from build123d import *

# Parameters (mm, degrees)
SKETCH_1_R          = 1.3
SKETCH_1_R_2        = 3
SKETCH_1_R_3        = 3.1
EXTRUDE_1_DEPTH     = 18
CUT_EXTRUDE_1_DEPTH = 39.778149269


with BuildPart() as part:
    # ｽｹｯﾁ1 → ﾎﾞｽ - 押し出し1 (new body)
    with BuildSketch(Plane.XY):
        with BuildLine():
            ThreePointArc((11.520520871, 18.842793666), (9.949769241, 24.020867845), (5.177628747, 21.470105609))
            ThreePointArc((5.177628747, 21.470105609), (0, 17.220935509), (-5.177628747, 21.470105609))
            ThreePointArc((-5.177628747, 21.470105609), (-9.949769241, 24.020867845), (-11.520520871, 18.842793666))
            ThreePointArc((-11.520520871, 18.842793666), (-12.177040277, 12.177040277), (-18.842793666, 11.520520871))
            ThreePointArc((-18.842793666, 11.520520871), (-24.020867845, 9.949769241), (-21.470105609, 5.177628747))
            ThreePointArc((-21.470105609, 5.177628747), (-17.220935509, 0), (-21.470105609, -5.177628747))
            ThreePointArc((-21.470105609, -5.177628747), (-24.020867845, -9.949769241), (-18.842793666, -11.520520871))
            ThreePointArc((-18.842793666, -11.520520871), (-12.177040277, -12.177040277), (-11.520520871, -18.842793666))
            ThreePointArc((-11.520520871, -18.842793666), (-9.949769241, -24.020867845), (-5.177628747, -21.470105609))
            ThreePointArc((-5.177628747, -21.470105609), (0, -17.220935509), (5.177628747, -21.470105609))
            ThreePointArc((5.177628747, -21.470105609), (9.949769241, -24.020867845), (11.520520871, -18.842793666))
            ThreePointArc((11.520520871, -18.842793666), (12.177040277, -12.177040277), (18.842793666, -11.520520871))
            ThreePointArc((18.842793666, -11.520520871), (24.020867845, -9.949769241), (21.470105609, -5.177628747))
            ThreePointArc((21.470105609, -5.177628747), (17.220935509, 0), (21.470105609, 5.177628747))
            ThreePointArc((21.470105609, 5.177628747), (24.020867845, 9.949769241), (18.842793666, 11.520520871))
            ThreePointArc((18.842793666, 11.520520871), (12.177040277, 12.177040277), (11.520520871, 18.842793666))
        make_face()
        with Locations((8.610377228, 20.787289482)):
            Circle(SKETCH_1_R, mode=Mode.SUBTRACT)
        with Locations((20.787289482, 8.610377228)):
            Circle(SKETCH_1_R, mode=Mode.SUBTRACT)
        with Locations((20.787289482, -8.610377228)):
            Circle(SKETCH_1_R, mode=Mode.SUBTRACT)
        with Locations((8.610377228, -20.787289482)):
            Circle(SKETCH_1_R, mode=Mode.SUBTRACT)
        with Locations((-8.610377228, -20.787289482)):
            Circle(SKETCH_1_R, mode=Mode.SUBTRACT)
        with Locations((-20.787289482, -8.610377228)):
            Circle(SKETCH_1_R, mode=Mode.SUBTRACT)
        with Locations((-20.787289482, 8.610377228)):
            Circle(SKETCH_1_R, mode=Mode.SUBTRACT)
        with Locations((-8.610377228, 20.787289482)):
            Circle(SKETCH_1_R, mode=Mode.SUBTRACT)
        with Locations((8.838834765, 8.838834765)):
            Circle(SKETCH_1_R, mode=Mode.SUBTRACT)
        with Locations((8.838834765, -8.838834765)):
            Circle(SKETCH_1_R, mode=Mode.SUBTRACT)
        with Locations((-8.838834765, -8.838834765)):
            Circle(SKETCH_1_R, mode=Mode.SUBTRACT)
        with Locations((-8.838834765, 8.838834765)):
            Circle(SKETCH_1_R, mode=Mode.SUBTRACT)
        with Locations((0, 6.5)):
            Circle(SKETCH_1_R, mode=Mode.SUBTRACT)
        with Locations((6.5, 0)):
            Circle(SKETCH_1_R, mode=Mode.SUBTRACT)
        with Locations((0, -6.5)):
            Circle(SKETCH_1_R, mode=Mode.SUBTRACT)
        with Locations((-6.5, 0)):
            Circle(SKETCH_1_R, mode=Mode.SUBTRACT)
        with Locations((0, 12.5)):
            Circle(SKETCH_1_R_2, mode=Mode.SUBTRACT)
        with Locations((12.5, 0)):
            Circle(SKETCH_1_R_2, mode=Mode.SUBTRACT)
        with Locations((0, -12.5)):
            Circle(SKETCH_1_R_2, mode=Mode.SUBTRACT)
        with Locations((-12.5, 0)):
            Circle(SKETCH_1_R_2, mode=Mode.SUBTRACT)
        Circle(SKETCH_1_R_3, mode=Mode.SUBTRACT)
    extrude(amount=EXTRUDE_1_DEPTH)

    # ｽｹｯﾁ2 → ｶｯﾄ - 押し出し1 (cut, through all)
    with BuildSketch(Plane.XY.offset(18)):
        with BuildLine():
            ThreePointArc((-15.5, 6e-09), (-12.499999997, 3), (-9.5, 0))
            ThreePointArc((-9.5, 0), (-9.355673654, 1.649657688), (-8.927079897, 3.249191362))
            ThreePointArc((-8.927079897, 3.249191362), (-10.72009733, 7.094329654), (-14.565235622, 5.301312222))
            ThreePointArc((-14.565235622, 5.301312222), (-15.264520171, 2.691546757), (-15.5, 6e-09))
        make_face()
        with BuildLine():
            ThreePointArc((-14.565235622, -5.301312222), (-10.72009733, -7.094329654), (-8.927079897, -3.249191362))
            ThreePointArc((-8.927079897, -3.249191362), (-9.355673654, -1.649657688), (-9.5, 0))
            ThreePointArc((-9.5, 0), (-12.500000003, -3), (-15.5, 6e-09))
            ThreePointArc((-15.5, 6e-09), (-15.264520172, -2.691546751), (-14.565235622, -5.301312222))
        make_face()
        with BuildLine():
            ThreePointArc((5.301312222, -14.565235622), (7.094329654, -10.72009733), (3.249191362, -8.927079897))
            ThreePointArc((3.249191362, -8.927079897), (1.649657689, -9.355673653), (3e-09, -9.5))
            ThreePointArc((3e-09, -9.5), (2.121320344, -10.378679657), (3, -12.5))
            ThreePointArc((3, -12.5), (2.121320344, -14.621320343), (1e-09, -15.5))
            ThreePointArc((1e-09, -15.5), (2.691546754, -15.264520172), (5.301312222, -14.565235622))
        make_face()
        with BuildLine():
            ThreePointArc((1e-09, -15.5), (-3, -12.499999999), (3e-09, -9.5))
            ThreePointArc((3e-09, -9.5), (-1.649657687, -9.355673654), (-3.249191362, -8.927079897))
            ThreePointArc((-3.249191362, -8.927079897), (-7.094329654, -10.72009733), (-5.301312222, -14.565235622))
            ThreePointArc((-5.301312222, -14.565235622), (-2.691546753, -15.264520172), (1e-09, -15.5))
        make_face()
        with BuildLine():
            ThreePointArc((15.5, 0), (12.499999993, -3), (9.5, 1.5e-08))
            ThreePointArc((9.5, 1.5e-08), (9.355673655, -1.649657681), (8.927079897, -3.249191362))
            ThreePointArc((8.927079897, -3.249191362), (10.72009733, -7.094329654), (14.565235622, -5.301312222))
            ThreePointArc((14.565235622, -5.301312222), (15.264520172, -2.691546754), (15.5, 0))
        make_face()
        with BuildLine():
            ThreePointArc((14.565235622, 5.301312222), (10.72009733, 7.094329654), (8.927079897, 3.249191362))
            ThreePointArc((8.927079897, 3.249191362), (9.355673652, 1.649657695), (9.5, 1.5e-08))
            ThreePointArc((9.5, 1.5e-08), (12.500000007, 3), (15.5, 0))
            ThreePointArc((15.5, 0), (15.264520172, 2.691546754), (14.565235622, 5.301312222))
        make_face()
        with BuildLine():
            ThreePointArc((-1.5e-08, 9.5), (1.649657681, 9.355673655), (3.249191362, 8.927079897))
            ThreePointArc((3.249191362, 8.927079897), (7.094329654, 10.72009733), (5.301312222, 14.565235622))
            ThreePointArc((5.301312222, 14.565235622), (2.691546753, 15.264520172), (-1e-09, 15.5))
            ThreePointArc((-1e-09, 15.5), (2.121320343, 14.621320344), (3, 12.5))
            ThreePointArc((3, 12.5), (2.121320338, 10.378679651), (-1.5e-08, 9.5))
        make_face()
        with BuildLine():
            ThreePointArc((-3.249191362, 8.927079897), (-1.649657695, 9.355673652), (-1.5e-08, 9.5))
            ThreePointArc((-1.5e-08, 9.5), (-3, 12.500000007), (-1e-09, 15.5))
            ThreePointArc((-1e-09, 15.5), (-2.691546754, 15.264520172), (-5.301312222, 14.565235622))
            ThreePointArc((-5.301312222, 14.565235622), (-7.094329654, 10.72009733), (-3.249191362, 8.927079897))
        make_face()
    extrude(amount=-CUT_EXTRUDE_1_DEPTH, mode=Mode.SUBTRACT)


solid = part.part
Geometry: final body of the model. Coordinates: model frame, mm. Give positions to 0.01 mm unless a question says otherwise; leave off trailing zeros. Loops run counter-clockwise (first coordinate to the right, second up) from the corner with the lowest first, then second, coordinate; pieces in that order, holes last. Notation, with made-up numbers: M -1.5,-7 L 14.5,-7 A22 ccw 14.5,4 Z; hole C 2.25,-32.75 d8. An arc over 180 degrees is marked long. Put each result on its own line as item: value. Start each with the question number.
1) Contact query for flat-ended pins moving along their axis: pin 1 (8 mm diameter, centred on x = 4.5, y = -18, fed in from -Z); pin 2 (4 mm diameter, centred on y = 11, z = 8.5, fed in from -X); pin 3 (1.6 mm diameter, centred on x = 8.61, y = 20.79, fed in from -Z); pin 4 (1 mm diameter, centred on y = -10, z = 4.5, fed in from -X). Output: stop coordinate, or through.
2) Ray query, line 1 along X through (y, z) = (21, 14); line 2 along Y through (x, z) = (2.5, 6.25); line 3 along X through (y, z) = (6, 8.75). Return the intervals inside material, ascending.
3) Cut plane A-A (y = -6.5). Output: boundary loops of the cut face in (x, z), then the cut area to 3 significant figures.
4) Pull-direction query (X, two-part tool) for faces 1 (the cylindrical face through (-8.01, -21.94, 8.87)), 2 (the cylindrical face through (17.22, -0.1, 8.87)), 3 (the flat face through (0, -5, 18)); classes: pulls with the +X half, pulls with the -X half, needs draft (parallel to the pull), parting line crosses it, or undercut.
5) Cut plane C-C (z = 10.75). Give the number of separate pieces and of enclosed holes in the cut face, then the cut area to 3 significant figures.
Verdict:
1. pin 1: z = 0
1. pin 2: x = -24.27
1. pin 3: through
1. pin 4: x = -24.17
2. line 1: -12.1 to -9.89, -7.33 to -5.06, 5.06 to 7.33, 9.89 to 12.1
2. line 2: -17.85 to -15.3, -9.17 to -1.83, 1.83 to 9.17, 15.3 to 17.85
2. line 3: -23.12 to -14.2, -9.29 to -1.2, 1.2 to 9.29, 14.2 to 23.12
3. outline: M -23.58,0 L -13.76,0 L -13.76,18 L -23.58,18 Z; M -9.73,0 L -1.3,0 L -1.3,18 L -9.73,18 Z; M 1.3,0 L 9.73,0 L 9.73,18 L 1.3,18 Z; M 13.76,0 L 23.58,0 L 23.58,18 L 13.76,18 Z
3. area: 657 mm2
4. face 1: undercut
4. face 2: pulls with the +X half
4. face 3: needs draft
5. separate pieces: 1
5. enclosed holes: 21
5. area: 979 mm2
